from build123d import *

# Parameters (mm, degrees)
CHANFRO1_SIZE         = 0.4
CORTE_EXTRUS_O1_DEPTH = 1.8
FILETE1_R             = 0.2


with BuildPart() as part:
    # Esboço4 → Revolução1 (revolve)
    with BuildSketch(Plane(origin=(0, 0, 0), x_dir=(0, 0, -1), z_dir=(1, 0, 0)), mode=Mode.PRIVATE) as revolu_o1_sk:
        Polygon((0, 4), (0, 0), (12, 0), (12, 2), (2.3, 2), (0.5, 4), align=None)
    revolve(revolu_o1_sk.sketch.rotate(Axis((0, 0, 0), (0, 0, -1)), 90), axis=Axis((0, 0, 0), (0, 0, -1)))

    # Chanfro1
    chanfro1_edges = [part.edges().sort_by_distance(p)[0] for p in [
        (-2, 0, -12),
    ]]
    chamfer(chanfro1_edges, length=CHANFRO1_SIZE)

    # Esboço5 → Corte-extrusão1 (cut)
    with BuildSketch(Plane.XY):
        Polygon((-1.25, -0.721687836), (0, -1.443375673), (1.25, -0.721687836), (1.25, 0.721687836), (0, 1.443375673), (-1.25, 0.721687836), align=None)
    extrude(amount=-CORTE_EXTRUS_O1_DEPTH, mode=Mode.SUBTRACT)

    # Corte-extrusão2 cone 1 section (through the dimple's axis) → Corte-extrusão2 (revolve, cut)
    with BuildSketch(Plane(origin=(0, 0, -1.8), x_dir=(0, -1, 0), z_dir=(1, 0, 0))):
        Polygon((0, 0), (1.25, 0), (0, 0.479830044), align=None)
    revolve(axis=Axis((0, 0, -1.8), (0, 0, -1)), mode=Mode.SUBTRACT)

    # Filete1
    filete1_edges = [part.edges().sort_by_distance(p)[0] for p in [
        (-2, 0, -2.3),
    ]]
    fillet(filete1_edges, radius=FILETE1_R)


solid = part.part
Work out the finished part from the listing and answer in its coordinate system (mm). A direction names the side the tool comes from. Give positions to 0.01 mm unless a question says otherwise; leave off trailing zeros. Loops run counter-clockwise (first coordinate to the right, second up) from the corner with the lowest first, then second, coordinate; pieces in that order, holes last. Notation, with made-up numbers: (44.25, 37) - (95.25, 37) arc R11 cw to (95.25, 47) - close; hole circle Ø5 at (71.25, 85.5). An arc over 180 degrees is marked (long way). Answer in a Markdown table with one row per item. Add a question column.
Q1. A tool of negligible diameter and unlimited length cuts with its end or side. For faces 1 (the flat face through (2, 0, 0)), 2 (the flat face through (-1.25, 0, -1)), 3 (the cylindrical face through (0, 2, -7)), from which of +Z, -Z, +X, -X, +Y, -Y can it reach the whole face along a straight path? Write none if from no direction.
Q2. Each of these flat-tipped pins is pushed along its axis until it touches: P1, Ø1, axis at x = -0.5, y = -3, coming from the -Z side; P2, Ø4, axis at y = -1.5, z = -2.5, coming from the +X side. Where does it stop, or does it pass through?
Q3. Determine the mould class of faces 4 (the flat face through (0.63, 1.08, -0.89)), 5 (the cylindrical face through (-0.867, 3.905, -0.246)), 6 (the flat face through (0, 0, -12)) for opening direction Y: released by +Y, released by -Y, zero draft, split by the parting line, or undercut.
Q4. The part is cut by section B-B (z = -4.25). Determine the outline of the cut face in (x, y), and give its area (3 significant figures).
Q5. The part is cut by section A-A (z = -1.5). Determine the outline of the cut face in (x, y).
Q6. Consider line 1 along Y through (x, z) = (0, -6); line 2 along X through (y, z) = (0.5, -0.75); line 3 along Z through (x, y) = (0.5, 3.5). Determine where each line is inside the solid, lowest interval first.
Solution:
| question | item | result |
|---|---|---|
| 1 | face 1 | +Z, +X, -X, +Y, -Y |
| 1 | face 2 | +Z |
| 1 | face 3 | -Z |
| 2 | P1 | stops at z = -1.81 |
| 2 | P2 | stops at x = 3.8 |
| 3 | face 4 | undercut |
| 3 | face 5 | split by the parting line |
| 3 | face 6 | zero draft |
| 4 | outline | circle Ø4 at (0, 0) |
| 4 | area | 12.6 mm² |
| 5 | outline | circle Ø5.78 at (0, 0); hole (-1.25, -0.72) - (0, -1.44) - (1.25, -0.72) - (1.25, 0.72) - (0, 1.44) - (-1.25, 0.72) - close |
| 6 | line 1 | y = -2 to 2 |
| 6 | line 2 | x = -3.69 to -1.25, 1.25 to 3.69 |
| 6 | line 3 | z = -0.92 to 0 |
